Geometry check sheet. Reference: the model listing, model coordinates, mm. Give positions to 0.01 mm unless a question says otherwise; leave off trailing zeros. Order: outer loops, then holes, each group sorted by start corner. A loop starts at its lowest first (then second) coordinate and runs counter-clockwise, first axis right, second up. Notation, with made-up numbers: M -10.5,-13 L 2.5,-13 A6 ccw 2.5,-9 Z; hole C 11.5,1 d6. An arc over 180 degrees is marked long. Answer as CSV lines item,"result".
from build123d import *

# Parameters (mm, degrees)
SKETCH_1_R          = 6.4
EXTRUDE_1_DEPTH     = 5
SKETCH_3_R          = 7.5
EXTRUDE_2_DEPTH     = 2
SKETCH_2_R          = 2
CUT_EXTRUDE_1_DEPTH = 8
FILLET_1_R          = 1
FILLET_2_R          = 1
FILLET_3_R          = 1


with BuildPart() as part:
    # 草图1 → 凸台-拉伸1 (new body)
    with BuildSketch(Plane(origin=(0, 0, 0), x_dir=(1, 0, 0), z_dir=(0, 1, 0))):
        Circle(SKETCH_1_R)
    extrude(amount=EXTRUDE_1_DEPTH)

    # 草图3 → 凸台-拉伸2 (add)
    with BuildSketch(Plane.XZ):
        Circle(SKETCH_3_R)
    extrude(amount=EXTRUDE_2_DEPTH)

    # 草图2 → 切除-拉伸1 (cut, through all)
    with BuildSketch(Plane(origin=(0, 5, 0), x_dir=(1, 0, 0), z_dir=(0, 1, 0))):
        Circle(SKETCH_2_R)
    extrude(amount=-CUT_EXTRUDE_1_DEPTH, mode=Mode.SUBTRACT)

    # 圆角1
    fillet_1_edges = [part.edges().sort_by_distance(p)[0] for p in [
        (-2, 5, 0),
        (-6.4, 5, 0),
    ]]
    fillet(fillet_1_edges, radius=FILLET_1_R)

    # 圆角2
    fillet_2_edges = [part.edges().sort_by_distance(p)[0] for p in [
        (-6.4, 0, 0),
    ]]
    fillet(fillet_2_edges, radius=FILLET_2_R)

    # 圆角3
    fillet_3_edges = [part.edges().sort_by_distance(p)[0] for p in [
        (-2, -2, 0),
    ]]
    fillet(fillet_3_edges, radius=FILLET_3_R)


solid = part.part
(1) Section check A-A on x = 0. Enter the section's corners in (y, z), then the cut area to 3 significant figures.
The answers:
outline,"M -2,-7.5 L 0,-7.5 L 0,-7.4 A1 cw 1,-6.4 L 4,-6.4 A1 ccw 5,-5.4 L 5,-3 A1 ccw 4,-2 L -1,-2 A1 ccw -2,-3 Z; M -2,3 A1 ccw -1,2 L 4,2 A1 ccw 5,3 L 5,5.4 A1 ccw 4,6.4 L 1,6.4 A1 cw 0,7.4 L 0,7.5 L -2,7.5 Z"
area,"65.1 mm2"
(2) Section check B-B on z = 0. Enter the section's corners in (x, y).
The answers:
outline,"M -7.5,-2 L -3,-2 A1 ccw -2,-1 L -2,4 A1 ccw -3,5 L -5.4,5 A1 ccw -6.4,4 L -6.4,1 A1 cw -7.4,0 L -7.5,0 Z; M 2,-1 A1 ccw 3,-2 L 7.5,-2 L 7.5,0 L 7.4,0 A1 cw 6.4,1 L 6.4,4 A1 ccw 5.4,5 L 3,5 A1 ccw 2,4 Z"
(3) Material ranges on line 1 (X direction, y = 1, z = 0); line 2 (X direction, y = 0.45, z = 0), recorded low to high.
The answers:
line 1,"x = -6.4 to -2, 2 to 6.4"
line 2,"x = -6.56 to -2, 2 to 6.56"
(4) Section check C-C on y = -0.25. Enter the section's corners in (x, z), then the cut area to 3 significant figures.
The answers:
outline,"C 0,0 d15; hole C 0,0 d4"
area,"164 mm2"
(5) Draft check along X on faces 1 (the face through (2.3, 5, 2.3)), 2 (the face through (-5.08, 2.48, 3.89)), 3 (the face through (0, 2, 2)). Enter one of: +X half, -X half, draft (parallel to the pull), parting line (faces both ways), or undercut.
The answers:
face 1,"draft"
face 2,"parting line"
face 3,"undercut"
(6) Gauge pin test, flat ends, axial feed: P1, Ø2, axis at y = 2.5, z = 3.5, coming from the -X side; P2, Ø2.5, axis at x = 0, z = 0, coming from the -Y side. Record the tip position at first contact, or that the pin passes through.
The answers:
P1,"stops at x = -5.89"
P2,"passes through"
(7) Section check D-D on y = 3. Enter the section's corners in (x, z), then the cut area to 3 significant figures.
The answers:
outline,"C 0,0 d12.8; hole C 0,0 d4"
area,"116 mm2"
